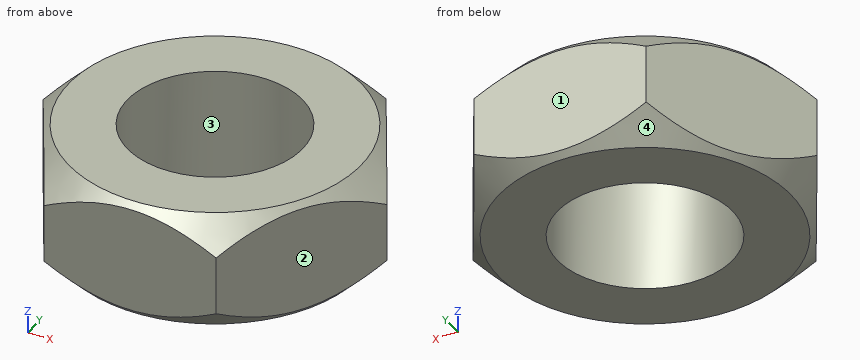
from build123d import *

# Parameters (mm, degrees)
SKETCH1_R           = 4.5
BOSS_EXTRUDE1_DEPTH = 3
SKETCH4_OUTSIDE_W   = 36.912
SKETCH4_OUTSIDE_H   = 34.5
SKETCH4_OUTSIDE_R   = 7.5
CUT_EXTRUDE1_DEPTH  = 6
CUT_EXTRUDE1_TAPER  = 45


with BuildPart() as part:
    # Sketch1 → Boss-Extrude1 (new body, symmetric)
    with BuildSketch(Plane.XY):
        Polygon((4.5, 7.794228634), (-4.5, 7.794228634), (-9, 0), (-4.5, -7.794228634), (4.5, -7.794228634), (9, 0), align=None)
        Circle(SKETCH1_R, mode=Mode.SUBTRACT)
    extrude(amount=BOSS_EXTRUDE1_DEPTH, both=True)

    # Sketch4 outside → Cut-Extrude1 (cut)
    with BuildSketch(Plane.XY.offset(3)):
        Rectangle(SKETCH4_OUTSIDE_W, SKETCH4_OUTSIDE_H)
        Circle(SKETCH4_OUTSIDE_R, mode=Mode.SUBTRACT)
    cut_extrude1 = extrude(amount=-CUT_EXTRUDE1_DEPTH, taper=CUT_EXTRUDE1_TAPER, mode=Mode.SUBTRACT)

    # Mirror1: Cut-Extrude1 across plane
    add(cut_extrude1.mirror(Plane.XY), mode=Mode.SUBTRACT)


solid = part.part
Geometry check sheet. Reference: the model listing, model coordinates, mm. Face numbers are marked on the shaded views. Round coordinates to 2 decimals unless told otherwise and drop trailing zeros. Order: outer loops, then holes, each group sorted by start corner. A loop starts at its lowest first (then second) coordinate and runs counter-clockwise, first axis right, second up. Notation, with made-up numbers: (-3.5, 63.25) - (33.5, 63.25) arc R17 cw to (33.5, 88.25) - close; hole circle Ø9 at (-25, 6). An arc over 180 degrees is marked (long way). One line per question, with ' | ' between items. Start each with the question number.
(1) Sectioned sample at A-A on x = 0. Record the cut outline in (y, z), and give its area (3 significant figures).
(2) Sectioned sample at B-B on z = -0.5. Record the cut outline in (x, y), and give its area (3 significant figures).
(3) Release check for a two-part mould opening along X. For the marked faces 1, 2, 3 and 4 record: released by +X, released by -X, zero draft, split by the parting line, or undercut.
(4) Thickness scan on L1, parallel to Y at x = 0, z = -0.8; L2, parallel to Y at x = -2.5, z = -0.25; L3, parallel to X at y = 1.75, z = 1.5. Record the ranges inside material, lowest first. Write a range as [from, to].
(5) Depth check by flat-ended pin: pin 1 Ø5.5 at (x, y) = (0, 0) entering from -Z. Enter the tip coordinate at first touch or a pass-through.
Conclusion:
1) outline: (-7.79, -2.71) - (-7.5, -3) - (-4.5, -3) - (-4.5, 3) - (-7.5, 3) - (-7.79, 2.71) - close; (4.5, -3) - (7.5, -3) - (7.79, -2.71) - (7.79, 2.71) - (7.5, 3) - (4.5, 3) - close | area: 39.4 mm2
2) outline: (-9, 0) - (-4.5, -7.79) - (4.5, -7.79) - (9, 0) - (4.5, 7.79) - (-4.5, 7.79) - close; hole circle Ø9 at (0, 0) | area: 147 mm2
3) face 1: zero draft | face 2: released by +X | face 3: undercut | face 4: split by the parting line
4) L1: y = [-7.79, -4.5], [4.5, 7.79] | L2: y = [-7.79, -3.74], [3.74, 7.79] | L3: x = [-7.99, -4.15], [4.15, 7.99]
5) pin 1: passes through
